Check sheet for the drawn part. Datum: minimum x, y, z corner. Units: mm. A direction names the side the tool comes from. Round coordinates to 2 decimals unless told otherwise and drop trailing zeros. Loops run counter-clockwise (first coordinate to the right, second up) from the corner with the lowest first, then second, coordinate; pieces in that order, holes last.
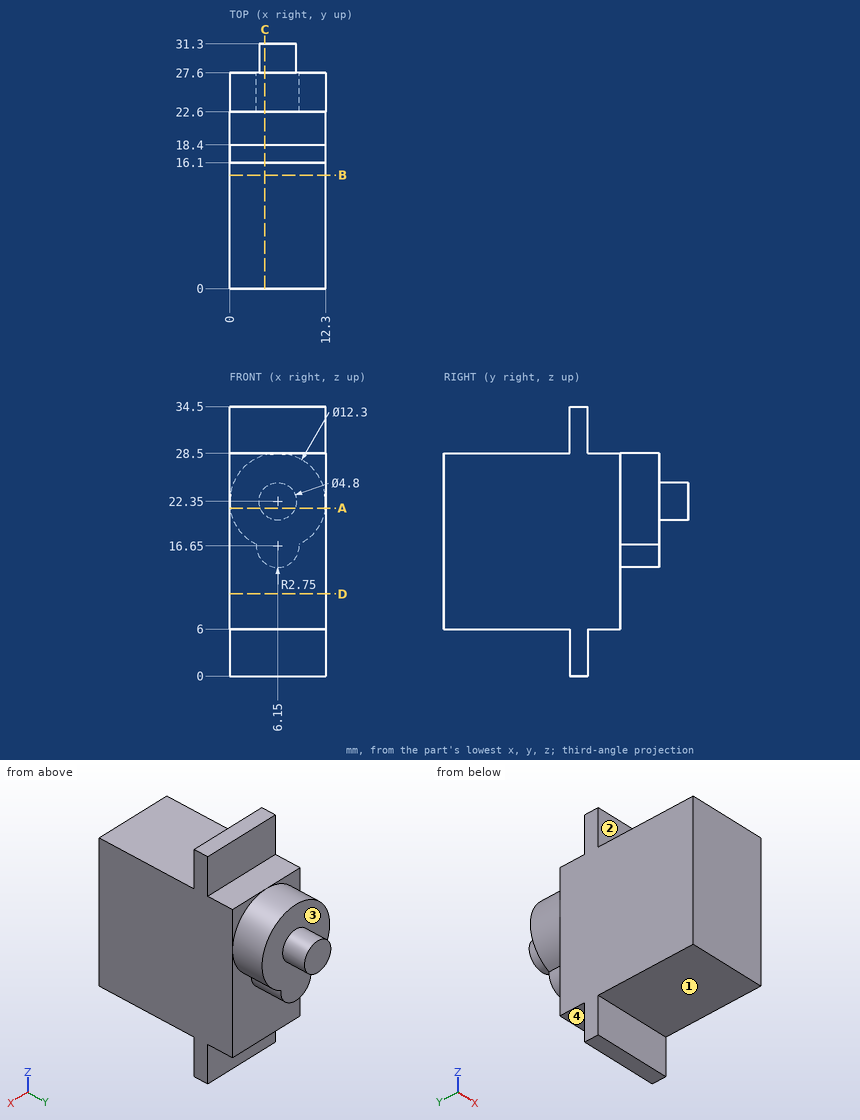
1) Gauge pin test, flat ends, axial feed: pin 1 (2 mm diameter, centred on x = 9, z = 9.5, fed in from +Y); pin 2 (3 mm diameter, centred on x = 6, z = 32, fed in from -Y); pin 3 (1.5 mm diameter, centred on y = 25.5, z = 20, fed in from +X); pin 4 (5 mm diameter, centred on x = 2, z = 4.5, fed in from -Y). Record the tip position at first contact, or that the pin passes through.
Report:
pin 1: stops at y = 22.6
pin 2: stops at y = 16.1
pin 3: stops at x = 12.09
pin 4: stops at y = 0
2) Access from +Z, -Z, +X, -X, +Y, -Y to the whole of each face (thin tool, end or side, straight path). Record for the marked faces 1, 2, 3 and 4.
Report:
face 1: -Z, +X, -X, -Y
face 2: +Z, +X, -X, -Y
face 3: +Y
face 4: -Z, +X, -X, +Y
3) Sectioned sample at B-B, the plane y = 14.5. Record the cut outline in (x, z), then the cut area to 3 significant figures.
Report:
outline: (0, 6) - (12.3, 6) - (12.3, 28.5) - (0, 28.5) - close
area: 277 mm2
4) Sectioned sample at D-D, the plane z = 10.5. Record the cut outline in (x, y), then the cut area to 3 significant figures.
Report:
outline: (0, 0) - (12.3, 0) - (12.3, 22.6) - (0, 22.6) - close
area: 278 mm2
5) Sectioned sample at C-C, the plane x = 4.5. Record the cut outline in (y, z), then the cut area to 3 significant figures.
Report:
outline: (0, 6) - (16.1, 6) - (16.1, 0) - (18.4, 0) - (18.4, 6) - (22.6, 6) - (22.6, 14.45) - (27.6, 14.45) - (27.6, 20.61) - (31.3, 20.61) - (31.3, 24.09) - (27.6, 24.09) - (27.6, 28.27) - (22.6, 28.27) - (22.6, 28.5) - (18.4, 28.5) - (18.4, 34.5) - (16.1, 34.5) - (16.1, 28.5) - (0, 28.5) - close
area: 618 mm2
6) Sectioned sample at A-A, the plane z = 21.5. Record the cut outline in (x, y).
Report:
outline: (0, 0) - (12.3, 0) - (12.3, 22.6) - (12.24, 22.6) - (12.24, 27.6) - (8.39, 27.6) - (8.39, 31.3) - (3.91, 31.3) - (3.91, 27.6) - (0.06, 27.6) - (0.06, 22.6) - (0, 22.6) - close
7) Scan lines: line 1 along Z through (x, y) = (8.5, 10); line 2 along Y through (x, z) = (2.25, 22.5); line 3 along Y through (x, z) = (2.5, 32). Record each from-to range of solid material in increasing order.
Report:
line 1: z = 6 to 28.5
line 2: y = 0 to 27.6
line 3: y = 16.1 to 18.4
